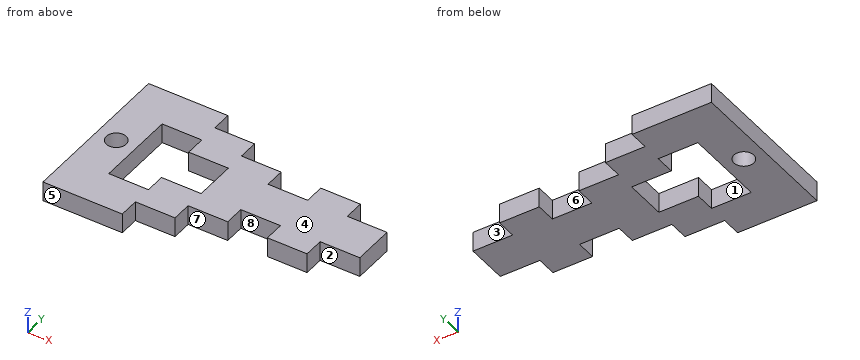
```python
from build123d import *

# Parameters (mm, degrees)
MODEL_R             = 1.5
BOSS_EXTRUDE1_DEPTH = 3


with BuildPart() as part:
    # Model → Boss-Extrude1 (new body)
    with BuildSketch(Plane.XY):
        Polygon((3258.106732125, 1248.388404039), (3264.106732125, 1248.388404039), (3264.106732125, 1245.388404039), (3264.106732125, 1242.138404039), (3258.106732125, 1242.138404039), (3258.106732125, 1239.138404039), (3252.106732125, 1239.138404039), (3252.106732125, 1242.138404039), (3246.106732125, 1242.138404039), (3246.106732125, 1239.138404039), (3240.106732125, 1239.138404039), (3240.106732125, 1236.138404039), (3234.106732125, 1236.138404039), (3234.106732125, 1233.138404039), (3228.106732125, 1233.138404039), (3222.106732125, 1233.138404039), (3222.106732125, 1245.388404039), (3222.106732125, 1257.388404039), (3228.106732125, 1257.388404039), (3234.106732125, 1257.388404039), (3234.106732125, 1254.388404039), (3240.106732125, 1254.388404039), (3240.106732125, 1251.388404039), (3246.106732125, 1251.388404039), (3246.106732125, 1248.388404039), (3252.106732125, 1248.388404039), (3252.106732125, 1251.388404039), (3258.106732125, 1251.388404039), align=None)
        with Locations((3225.106732125, 1245.388404039)):
            Circle(MODEL_R, mode=Mode.SUBTRACT)
        Polygon((3240.106732125, 1248.388404039), (3234.106732125, 1248.388404039), (3234.106732125, 1251.388404039), (3228.106732125, 1251.388404039), (3228.106732125, 1245.388404039), (3228.106732125, 1239.138404039), (3234.106732125, 1239.138404039), (3234.106732125, 1242.138404039), (3240.106732125, 1242.138404039), align=None, mode=Mode.SUBTRACT)
    extrude(amount=BOSS_EXTRUDE1_DEPTH)


solid = part.part
```
CAD build for the part. Positions are in the model's coordinates, mm. Face numbers are marked on the shaded views. A direction names the side the tool comes from. Coordinates: 2 decimals unless noted, no trailing zeros. Order: outer loops, then holes, each group sorted by start corner. A loop starts at its lowest first (then second) coordinate and runs counter-clockwise, first axis right, second up. Notation, with made-up numbers: (56, 28.25) - (74, 28.25) arc R18 ccw to (74, 36.25) - close; hole circle Ø8 at (3.25, -11.75). An arc over 180 degrees is marked (long way). Use a Markdown table: item, result. Add a question column.
(1) Saw through at B-B (x = 3239.5). Give the cut face in (y, z).
(2) Saw through at A-A (y = 1239.75). Give the cut face in (x, z).
(3) Pull direction X, two halves, no side cores. Call the marked faces 6, 7 and 8: +X half, -X half, draft (parallel to the pull), parting line (faces both ways), or undercut.
(4) Saw through at D-D (x = 3260). Give the cut face in (y, z), then the cut area to 4 significant figures.
(5) Saw through at C-C (z = 1.6). Count the separate pieces of the cut face and the enclosed holes in it, then the cut area to 3 significant figures.
(6) Drill centre lines: line 1 along X through (y, z) = (1240, 1); line 2 along Y through (x, z) = (3230.5, 2.8); line 3 along Y through (x, z) = (3239, 0.85). Where is each one in solid material? Low to high. Write a range as [from, to].
(7) Which spindle directions (+Z, -Z, +X, -X, +Y, -Y) get a long thin tool onto all of the face, cutting with end or side? Do the marked faces 1, 2, 3, 4 and 5. Say none if no direction does.
(8) Flat gauge pins, fed straight in: pin 1 (0.9 mm diameter, centred on x = 3244, z = 1.5, fed in from -Y); pin 2 (1.5 mm diameter, centred on x = 3236, z = 0.5, fed in from +Y); pin 3 (0.9 mm diameter, centred on x = 3244, z = 1, fed in from +Y); pin 4 (2.5 mm diameter, centred on x = 3225.11, y = 1245.39, fed in from +Z). Where does each tip first touch, or does it go through?
Solved:
| question | item | result |
|---|---|---|
| 1 | outline | (1236.14, 0) - (1242.14, 0) - (1242.14, 3) - (1236.14, 3) - close; (1248.39, 0) - (1254.39, 0) - (1254.39, 3) - (1248.39, 3) - close |
| 2 | outline | (3222.11, 0) - (3228.11, 0) - (3228.11, 3) - (3222.11, 3) - close; (3234.11, 0) - (3246.11, 0) - (3246.11, 3) - (3234.11, 3) - close; (3252.11, 0) - (3258.11, 0) - (3258.11, 3) - (3252.11, 3) - close |
| 3 | face 6 | undercut |
| 3 | face 7 | draft |
| 3 | face 8 | undercut |
| 4 | outline | (1242.14, 0) - (1248.39, 0) - (1248.39, 3) - (1242.14, 3) - close |
| 4 | area | 18.75 mm² |
| 5 | separate pieces | 1 |
| 5 | enclosed holes | 2 |
| 5 | area | 504 mm² |
| 6 | line 1 | x = [3222.11, 3228.11], [3234.11, 3246.11], [3252.11, 3258.11] |
| 6 | line 2 | y = [1233.14, 1239.14], [1251.39, 1257.39] |
| 6 | line 3 | y = [1236.14, 1242.14], [1248.39, 1254.39] |
| 7 | face 1 | +Z, -Z |
| 7 | face 2 | +Z, -Z, +X, -Y |
| 7 | face 3 | +Z, -Z, +X, +Y |
| 7 | face 4 | +Z, +X, -X, +Y, -Y |
| 7 | face 5 | +Z, -Z, +X, -X, -Y |
| 8 | pin 1 | stops at y = 1239.14 |
| 8 | pin 2 | stops at y = 1254.39 |
| 8 | pin 3 | stops at y = 1251.39 |
| 8 | pin 4 | passes through |
